from build123d import *

# Parameters (mm, degrees)
SKETCH1_W           = 150
SKETCH1_H           = 75
BOSS_EXTRUDE1_DEPTH = 5
SKETCH2_W           = 75
SKETCH2_H           = 50
BOSS_EXTRUDE2_DEPTH = 2
CHAMFER1_SIZE       = 20


with BuildPart() as part:
    # Sketch1 → Boss-Extrude1 (new body)
    with BuildSketch(Plane(origin=(0, 0, 0), x_dir=(1, 0, 0), z_dir=(0, 1, 0))):
        Rectangle(SKETCH1_W, SKETCH1_H)
    extrude(amount=BOSS_EXTRUDE1_DEPTH)

    # Sketch2 → Boss-Extrude2 (add)
    with BuildSketch(Plane.ZY.offset(75)):
        with Locations((0, 25)):
            Rectangle(SKETCH2_W, SKETCH2_H)
    boss_extrude2 = extrude(amount=BOSS_EXTRUDE2_DEPTH)

    # Mirror1: Boss-Extrude2 across plane
    add(boss_extrude2.mirror(Plane(origin=(0, 0, 0), x_dir=(0, 0, 1), z_dir=(1, 0, 0))))

    # Chamfer1
    chamfer1_edges = [part.edges().sort_by_distance(p)[0] for p in [
        (76, 50, -37.5),
        (76, 50, 37.5),
    ]]
    chamfer(chamfer1_edges, length=CHAMFER1_SIZE)


solid = part.part
Input: part model. Units: mm. Frame: model coordinates. A direction names the side the tool comes from. Coordinates: 2 decimals unless noted, no trailing zeros. Order: outer loops, then holes, each group sorted by start corner. A loop starts at its lowest first (then second) coordinate and runs counter-clockwise, first axis right, second up.
1. Draft query along X for faces 4 (the flat face through (77, 25, -1)), 5 (the flat face through (-1, 0, -1)), 6 (the flat face through (75, 28, -1)). Return one class per face: +X half, -X half, draft (parallel to the pull), parting line (faces both ways), or undercut.
Checked values:
face 4: +X half
face 5: draft
face 6: undercut
2. Cut plane D-D, the plane z = -28. Return loops of the section in (x, y), plus the area to 3 significant figures.
Checked values:
outline: (-77, 0) - (77, 0) - (77, 39.5) - (75, 39.5) - (75, 5) - (-75, 5) - (-75, 50) - (-77, 50) - close
area: 929 mm2
3. Access query for faces 1 (the flat face through (76, 40.1, -27.4)), 2 (the flat face through (-1, 5, -1)), 3 (the flat face through (76, 40.1, 27.4)). Directions: +Z, -Z, +X, -X, +Y, -Y. A direction counts if a zero-diameter tool reaches every point of the face in a straight line with its end or side. Return the directions, or none.
Checked values:
face 1: -Z, +X, +Y
face 2: +Z, -Z, +Y
face 3: +Z, +X, +Y
4. Cut plane A-A, the plane y = 28. Return loops of the section in (x, z).
Checked values:
outline: (-77, -37.5) - (-75, -37.5) - (-75, 37.5) - (-77, 37.5) - close; (75, -37.5) - (77, -37.5) - (77, 37.5) - (75, 37.5) - close
5. Ray query, line 1 along X through (y, z) = (31.5, 21.5); line 2 along X through (y, z) = (41.5, 32); line 3 along Y through (x, z) = (60, 18). Return the intervals inside material, ascending.
Checked values:
line 1: x = -77 to -75, 75 to 77
line 2: x = -77 to -75
line 3: y = 0 to 5
6. Contact query for flat-ended pins moving along their axis: P1, Ø22.5, axis at x = -7.5, z = 15, coming from the +Y side; P2, Ø3, axis at y = 41, z = 28.5, coming from the +X side. Output: stop coordinate, or through.
Checked values:
P1: stops at y = 5
P2: stops at x = 77
7. Cut plane B-B, the plane z = -12. Return loops of the section in (x, y), plus the area to 3 significant figures.
Checked values:
outline: (-77, 0) - (77, 0) - (77, 50) - (75, 50) - (75, 5) - (-75, 5) - (-75, 50) - (-77, 50) - close
area: 950 mm2
8. Cut plane C-C, the plane y = 45. Return loops of the section in (x, z), plus the area to 3 significant figures.
Checked values:
outline: (-77, -37.5) - (-75, -37.5) - (-75, 37.5) - (-77, 37.5) - close; (75, -22.5) - (77, -22.5) - (77, 22.5) - (75, 22.5) - close
area: 240 mm2
